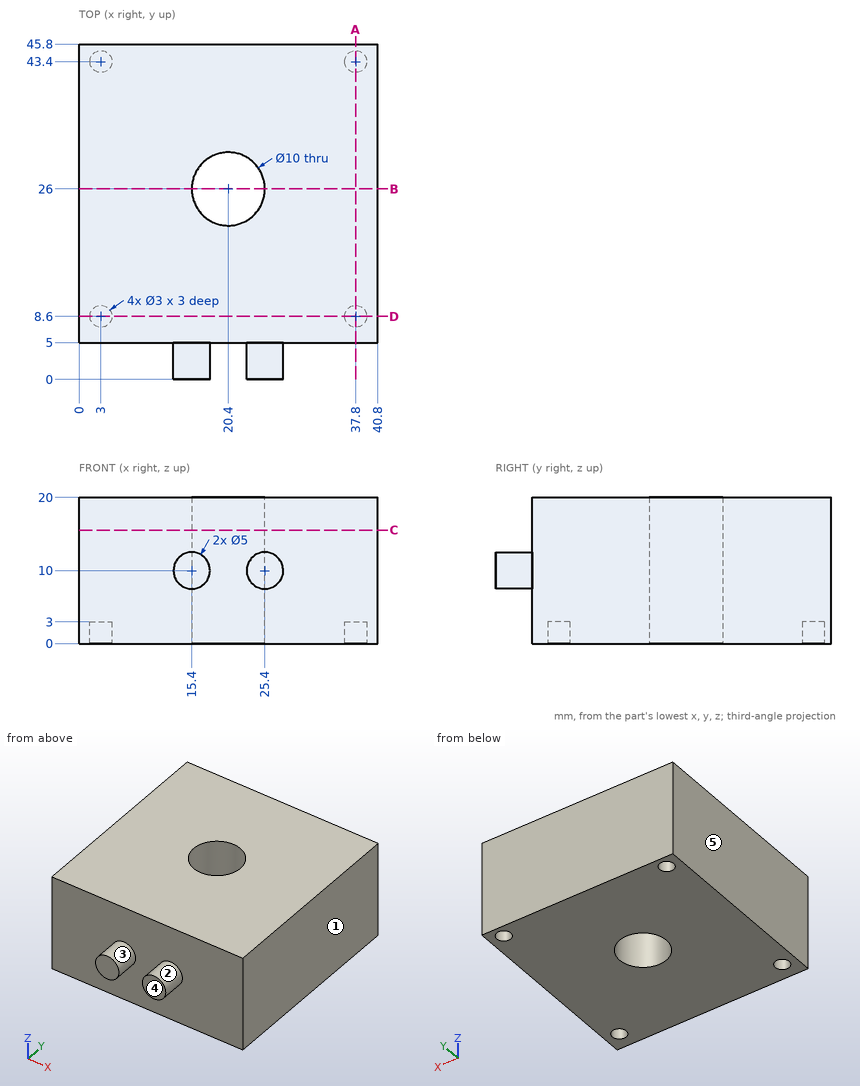
Drawing for the job (mm, zero at the part's lowest x, y, z). A direction names the side the tool comes from. Give positions to 0.01 mm unless a question says otherwise; leave off trailing zeros. Order: outer loops, then holes, each group sorted by start corner. A loop starts at its lowest first (then second) coordinate and runs counter-clockwise, first axis right, second up. Notation, with made-up numbers: M -8,16 L 16,16 A9 cw 16,29 Z; hole C 74,-12.75 d6. An arc over 180 degrees is marked long. Use a Markdown table: item, result. Add a question column.
(1) Saw through at D-D, the plane y = 8.6. Give the cut face in (x, z).
(2) 3-axis set-ups, long thin cutter, end or side, ignore diameter. For the marked faces 1 and 2: which of +Z, -Z, +X, -X, +Y, -Y reach the whole face in a straight line?
(3) Saw through at C-C, the plane z = 15.5. Give the cut face in (x, y), and give its area (3 significant figures).
(4) Drop a flat-ended pin along its axis: P1, Ø0.9, axis at x = 38.5, y = 44, coming from the -Z side. Give the stop position or say it passes through.
(5) Mould opens along X. For the marked faces 3, 4 and 5 say: +X half, -X half, draft (parallel to the pull), parting line (faces both ways), or undercut.
(6) Probe line 1 along Y through (x, z) = (37.8, 2.05); line 2 along Y through (x, z) = (20.4, 15.75); line 3 along Y through (x, z) = (37, 18.75). List the from-to ranges inside material, lowest first. Write a range as [from, to].
(7) Saw through at B-B, the plane y = 26. Give the cut face in (x, z).
(8) Saw through at A-A, the plane x = 37.8. Give the cut face in (y, z).
Answer key:
| question | item | result |
|---|---|---|
| 1 | outline | M 0,0 L 1.5,0 L 1.5,3 L 4.5,3 L 4.5,0 L 36.3,0 L 36.3,3 L 39.3,3 L 39.3,0 L 40.8,0 L 40.8,20 L 0,20 Z |
| 2 | face 1 | +Z, -Z, +X, +Y, -Y |
| 2 | face 2 | -Y |
| 3 | outline | M 0,5 L 40.8,5 L 40.8,45.8 L 0,45.8 Z; hole C 20.4,26 d10 |
| 3 | area | 1,590 mm^2 |
| 4 | P1 | z = 3 |
| 5 | face 3 | undercut |
| 5 | face 4 | draft |
| 5 | face 5 | -X half |
| 6 | line 1 | [5, 7.1], [10.1, 41.9], [44.9, 45.8] |
| 6 | line 2 | [5, 21], [31, 45.8] |
| 6 | line 3 | [5, 45.8] |
| 7 | outline | M 0,0 L 15.4,0 L 15.4,20 L 0,20 Z; M 25.4,0 L 40.8,0 L 40.8,20 L 25.4,20 Z |
| 8 | outline | M 5,0 L 7.1,0 L 7.1,3 L 10.1,3 L 10.1,0 L 41.9,0 L 41.9,3 L 44.9,3 L 44.9,0 L 45.8,0 L 45.8,20 L 5,20 Z |
